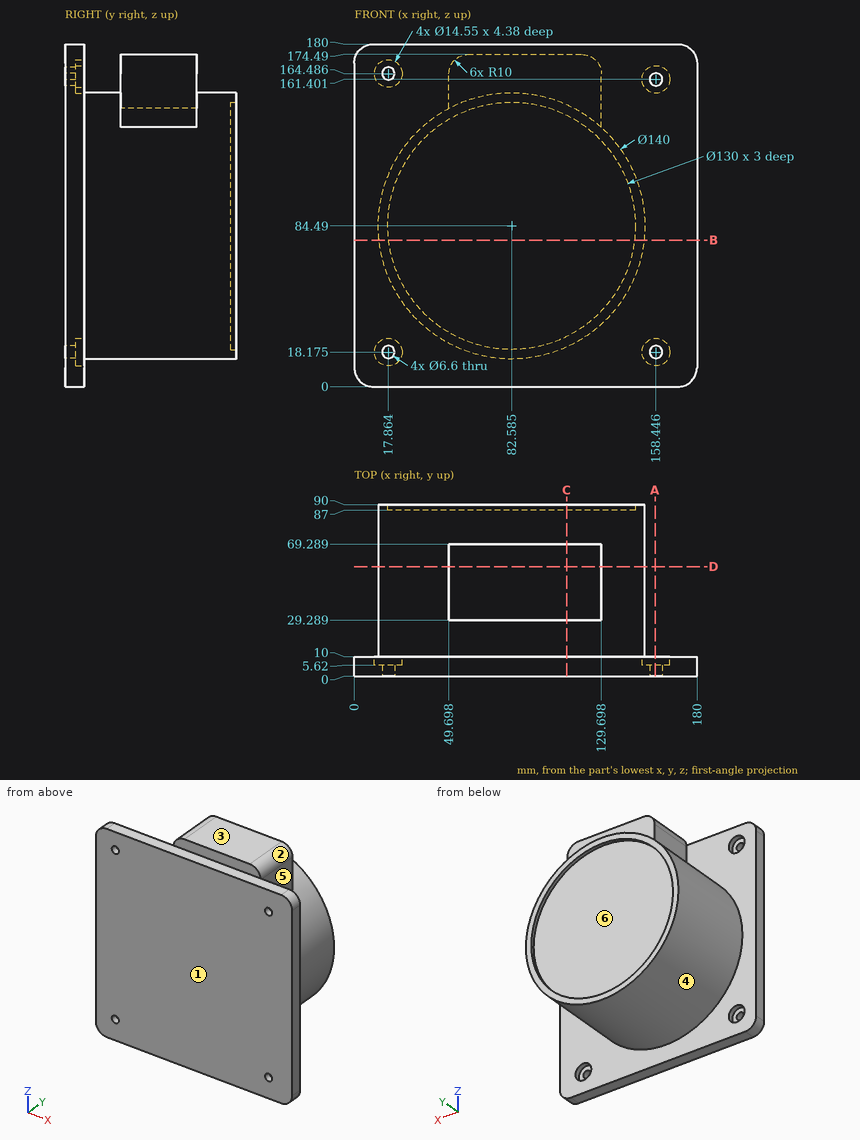
For this review, use the dimensioned drawing (mm, ordinates from the lowest corner) and the shaded views. A direction names the side the tool comes from. Give positions to 0.01 mm unless a question says otherwise; leave off trailing zeros. Order: outer loops, then holes, each group sorted by start corner. A loop starts at its lowest first (then second) coordinate and runs counter-clockwise, first axis right, second up. Notation, with made-up numbers: M 14,75 L 21,75 A9 ccw 21,81 Z; hole C 8,49.5 d2. An arc over 180 degrees is marked long. Use one line per item in the form item = value. Start each with the question number.
Item 1: We need section B-B on z = 77. Give the boundary of the cut face in (x, y).
Item 2: The part is to be moulded in two halves that separate along X. For the marked faces 4, 5 and 6, say which applies: pulls with the +X half, pulls with the -X half, needs draft (parallel to the pull), parting line crosses it, or undercut.
Item 3: To check wall thickness, follow line 1 along Y through (x, z) = (11, 31); line 2 along Y through (x, z) = (61.5, 28); line 3 along X through (y, z) = (65, 58.5). State the ranges of each line that lie inside material, in increasing order. Write a range as from..to.
Item 4: We need section A-A on x = 158. Give the boundary of the cut face in (y, z) (1 decimal).
Item 5: For the marked faces 1, 2 and 3, list the 3-axis set-ups (+Z, -Z, +X, -X, +Y, -Y) from which the entire face can be reached by the end or side of a thin tool; tool diameter is ignored.
Item 6: We need section C-C on x = 111.5. Give the boundary of the cut face in (y, z) (1 decimal).
Item 7: We need section D-D on y = 57.5. Give the boundary of the cut face in (x, z) (1 decimal), plus the area to 3 significant figures.
Item 8: Insertion check: pin 1 Ø13 at (x, z) = (158.45, 18.18) entering from +Y; pin 2 Ø7.5 at (x, z) = (157, 158) entering from +Y; pin 3 Ø4 at (y, z) = (70, 77) entering from -X. Each pin has a flat end and moves straight along its axis. Give the tip position at first contact, or say it passes through.
Completed:
q1.outline = M 0,0 L 180,0 L 180,10 L 152.18,10 L 152.18,90 L 147.15,90 L 147.15,87 L 18.02,87 L 18.02,90 L 12.99,90 L 12.99,10 L 0,10 Z
q2.face_4 = parting line crosses it
q2.face_5 = pulls with the +X half
q2.face_6 = undercut
q3.line_1 = 0..10
q3.line_2 = 0..87
q3.line_3 = 17.59..147.58
q4.outline = M 0,0 L 10,0 L 10,10.9 L 5.6,10.9 L 5.6,14.9 L 0,14.9 Z; M 0,21.4 L 5.6,21.4 L 5.6,25.4 L 10,25.4 L 10,154.1 L 5.6,154.1 L 5.6,158.1 L 0,158.1 Z; M 0,164.7 L 5.6,164.7 L 5.6,168.7 L 10,168.7 L 10,180 L 0,180 Z
q5.face_1 = +Z, -Z, +X, -X, -Y
q5.face_2 = +Z, +X, +Y
q5.face_3 = +Z, +X, -X, +Y
q6.outline = M 0,0 L 10,0 L 10,20.7 L 90,20.7 L 90,26.3 L 87,26.3 L 87,142.7 L 90,142.7 L 90,148.2 L 69.3,148.2 L 69.3,174.5 L 29.3,174.5 L 29.3,148.2 L 10,148.2 L 10,180 L 0,180 Z
q7.outline = M 49.7,146.3 A70 ccw long 129.7,136.3 L 129.7,164.5 A10 ccw 119.7,174.5 L 59.7,174.5 A10 ccw 49.7,164.5 Z
q7.area = 17,300 mm²
q8.pin_1 = 5.62
q8.pin_2 = 10
q8.pin_3 = 12.8
